```python
from build123d import *

# Parameters (mm, degrees)
F1_DEPTH = 21.43125
F2_R     = 9.525
F3_DEPTH = 50.8
F6_DEPTH = 42.8635
F7_DEPTH = 61.9829719698


with BuildPart() as f1:
    # F0 (on Right) → F1 (new body, symmetric)
    with BuildSketch(Plane.YZ):
        Polygon((-152.4, 69.85), (-152.4, 0), (152.4, 0), (152.4, 19.05), align=None)
    extrude(amount=F1_DEPTH, both=True)

    # F2 (on face) → F3 (cut)
    with BuildSketch(Plane.XZ.offset(152.4)):
        with Locations((0, 34.925)):
            Circle(F2_R)
    extrude(amount=-F3_DEPTH, mode=Mode.SUBTRACT)

    # F4 (on face) → F6 (cut, through all)
    with BuildSketch(Plane.YZ.offset(21.43125)):
        with BuildLine():
            Line((-152.4, 69.85), (-152.4, 59.5187321305))
            add(Edge.make_bspline(
                [(-152.4, 59.5187321305), (-142.2583344868, 61.4276814743), (-116.1526932903, 66.3415042155), (-72.0639469007, 40.8688743493), (-45.1030433178, 25.2919942141)],
                knots=[0, 0, 0, 0, 0.3884855935, 1, 1, 1, 1], degree=3))
            Line((-45.1030433178, 25.2919942141), (152.4, 14.1683043912))
            Line((152.4, 14.1683043912), (152.4, 19.05))
            Line((152.4, 19.05), (-152.4, 69.85))
        make_face()
    extrude(amount=-F6_DEPTH, mode=Mode.SUBTRACT)

    # F5 (on face) → F7 (intersect, through all)
    with BuildSketch(Plane(origin=(0, 0, 0), x_dir=(1, 0, 0), z_dir=(0, 0, -1))):
        with BuildLine():
            Line((-21.43125, 152.4), (-21.43125, 88.3942618966))
            add(Edge.make_bspline(
                [(-21.43125, 88.3942618966), (-16.4613031807, 79.4460650051), (-1.6409073495, 52.762515919), (-13.5294629941, -27.8924381707), (-21.43125, -81.5001502633)],
                knots=[0, 0, 0, 0, 0.3353450796, 1, 1, 1, 1], degree=3))
            Line((-21.43125, -81.5001502633), (-5.206305068, -152.4))
            Line((-5.206305068, -152.4), (5.206305068, -152.4))
            Line((5.206305068, -152.4), (21.43125, -81.5001502633))
            add(Edge.make_bspline(
                [(21.43125, 88.3942618966), (16.4613031807, 79.4460650051), (1.6409073495, 52.762515919), (13.5294629941, -27.8924381707), (21.43125, -81.5001502633)],
                knots=[0, 0, 0, 0, 0.3353450796, 1, 1, 1, 1], degree=3))
            Line((21.43125, 88.3942618966), (21.43125, 152.4))
            Line((21.43125, 152.4), (-21.43125, 152.4))
        make_face()
    extrude(amount=-F7_DEPTH, mode=Mode.INTERSECT)


solid = f1.part
```
Input: part model. Units: mm. Frame: model coordinates. A direction names the side the tool comes from. Coordinates: 2 decimals unless noted, no trailing zeros. Write each loop counter-clockwise with the first axis right and the second up, starting at its lowest first coordinate (ties: lowest second). Pieces come first, ordered by that corner, then holes.
1) Section A-A on y = 106.5. Output: boundary loops of the cut face in (x, z).
2) Material intervals for line 1 along Z through (x, y) = (0, -133); line 2 along Z through (x, y) = (0, -124); line 3 along Z through (x, y) = (16.5, 49.5), sorted ascending.
3) Mould query, pull axis Z, two halves, no side actions, for faces 1 (the flat face through (-21.431, -121, 31)), 2 (the flat face through (0, -101.6, 35)), 3 (the flat face through (0.3, 52.266, 19.808)). Classes: pulls with the +Z half, pulls with the -Z half, needs draft (parallel to the pull), parting line crosses it, or undercut.
4) Pin query (flat end, axial travel): pin 1 Ø5.5 at (x, z) = (3, 37) entering from -Y; pin 2 Ø10 at (x, y) = (-7.5, 19.5) entering from +Z; pin 3 Ø3 at (y, z) = (49, 7.5) entering from -X. Return the tip coordinate at first contact, or that it passes through.
5) Set-up query: faces 4 (the flat face through (0, -2, 0)), 5 (the cylindrical face through (-1.24, -127.36, 44.37)). Return all of +Z, -Z, +X, -X, +Y, -Y with unobstructed straight access to the full face (end or side cutting, diameter ignored); none if empty.
Check result:
1. outline: (-15.71, 0) - (15.71, 0) - (15.71, 16.75) - (-15.71, 16.75) - close
2. line 1: z = 0 to 25.4, 44.45 to 61.97
2. line 2: z = 0 to 25.4, 44.45 to 61.46
2. line 3: z = 0 to 19.96
3. face 1: needs draft
3. face 2: undercut
3. face 3: pulls with the +Z half
4. pin 1: stops at y = -101.6
4. pin 2: stops at z = 21.94
4. pin 3: stops at x = -16.92
5. face 4: -Z, +X, -X, +Y, -Y
5. face 5: -Y
